Part model, mm, in its own coordinate system. Coordinates: 2 decimals unless noted, no trailing zeros. Order: outer loops, then holes, each group sorted by start corner. A loop starts at its lowest first (then second) coordinate and runs counter-clockwise, first axis right, second up.
```python
from build123d import *

# Parameters (mm, degrees)
BOSS_EXTRUDE1_DEPTH = 1.5875
SKETCH2_R           = 1.651
CUT_EXTRUDE1_DEPTH  = 3.175


with BuildPart() as part:
    # Sketch1 → Boss-Extrude1 (new, symmetric)
    with BuildSketch(Plane(origin=(0, 0, 0), x_dir=(1, 0, 0), z_dir=(0, 1, 0))):
        Polygon((66.675, 19.05), (88.672045256, 19.05), (66.675, -19.05), (-66.675, -19.05), (-66.675, 19.05), align=None)
    extrude(amount=BOSS_EXTRUDE1_DEPTH, both=True)

    # Sketch2 → Cut-Extrude1 (cut)
    with BuildSketch(Plane(origin=(0, 1.5875, 0), x_dir=(1, 0, 0), z_dir=(0, 1, 0))):
        with Locations(Location((-57.023, 9.525, 0), (0, 0, 270))):
            Circle(SKETCH2_R)
        with Locations(Location((-57.023, -9.525, 0), (0, 0, 270))):
            Circle(SKETCH2_R)
        with Locations(Location((44.323, -9.525, 0), (0, 0, 270))):
            Circle(SKETCH2_R)
        with Locations(Location((44.323, 9.525, 0), (0, 0, 270))):
            Circle(SKETCH2_R)
    extrude(amount=-CUT_EXTRUDE1_DEPTH, mode=Mode.SUBTRACT)


solid = part.part
```
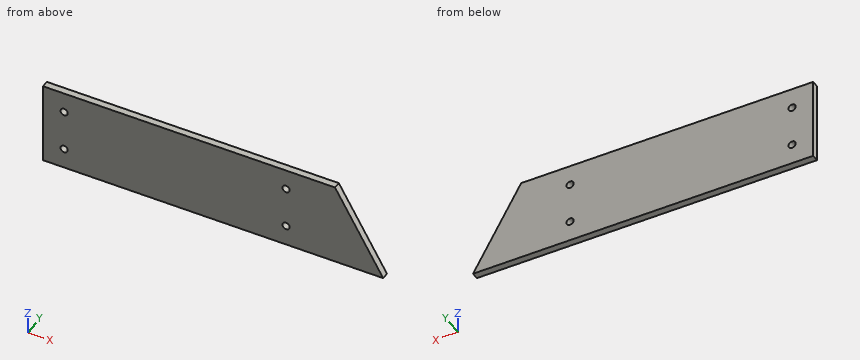
(1) Drop flat-ended pins along their axis: pin 1 (4.5 mm diameter, centred on x = -57.023, z = 9.525, fed in from -Y); pin 2 (2 mm diameter, centred on x = 44.323, z = 9.525, fed in from -Y). Give the stop position or say it passes through.
(2) Slice it at B-B, the plane z = 0. Give the cut face in (x, y) (1 decimal).
(3) Probe line 1 (Z direction, x = -58, y = 1.45); line 2 (X direction, y = 0.05, z = -0.5) (3 decimals); line 3 (X direction, y = -0.5, z = 4) (3 decimals). List the from-to ranges inside material, lowest first.
(4) Slice it at A-A, the plane y = -0.8. Give the cut face in (x, z) (3 decimals), then the cut area to 3 significant figures.
(5) Slice it at C-C, the plane x = 68. Give the cut face in (y, z).
Here are the results:
1. pin 1: stops at y = -1.59
1. pin 2: passes through
2. outline: (-66.7, -1.6) - (77.7, -1.6) - (77.7, 1.6) - (-66.7, 1.6) - close
3. line 1: z = -19.05 to -10.86, -8.19 to 8.19, 10.86 to 19.05
3. line 2: x = -66.675 to 77.962
3. line 3: x = -66.675 to 75.364
4. outline: (-66.675, -19.05) - (88.672, -19.05) - (66.675, 19.05) - (-66.675, 19.05) - close; hole circle Ø3.302 at (-57.023, -9.525); hole circle Ø3.302 at (-57.023, 9.525); hole circle Ø3.302 at (44.323, -9.525); hole circle Ø3.302 at (44.323, 9.525)
4. area: 5,470 mm2
5. outline: (-1.59, -19.05) - (1.59, -19.05) - (1.59, 16.76) - (-1.59, 16.76) - close
